Design review of the part built by this model. Coordinates are the model's own, in mm. A direction names the side the tool comes from. Coordinates: 2 decimals unless noted, no trailing zeros. Write each loop counter-clockwise with the first axis right and the second up, starting at its lowest first coordinate (ties: lowest second). Pieces come first, ordered by that corner, then holes.
Q1. For L1, parallel to X at y = 1.3, z = 9; L2, parallel to Z at x = -13, y = -3.75; L3, parallel to X at y = -0.05, z = 9, list the stretches that pass through material, from the lowest coordinate up.
Q2. For faces 1 (the flat face through (8, -4, -12.5)), 2 (the flat face through (0, 0, 0)), 3 (the flat face through (5.5, 1, -9)), list the 3-axis set-ups (+Z, -Z, +X, -X, +Y, -Y) from which the entire face can be reached by the end or side of a thin tool; tool diameter is ignored.
Q3. Take a section at A-A, the plane x = 0. Write out the cut boundary in (y, z).
Q4. The part is to be moulded in two halves that separate along Z. For faces 4 (the cylindrical face through (0.481, 0.816, 10.526)), 5 (the flat face through (0, 1, -2.25)), 6 (the flat face through (0, 2, 0)), say which applies: released by +Z, released by -Z, zero draft, split by the parting line, or undercut.
Q5. Take a section at D-D, the plane y = -4.75. Write out the cut boundary in (x, z).
Q6. Take a section at B-B, the plane y = 0.5. Write out the cut boundary in (x, z), plus the area to 3 significant figures.
Q7. Take a section at C-C, the plane x = -9. Write out the cut boundary in (y, z).
Q8. For pin 1 Ø0.6 at (x, y) = (1, 1) entering from -Z; pin 2 Ø4 at (x, z) = (18, 0.5) entering from -Y; pin 3 Ø5 at (y, z) = (-1.5, -10) entering from -X, all flat-tipped, find the tip position at first contact; note any pin that passes through.
from build123d import *

# Parameters (mm, degrees)
BOSS_EXTRUDE1_DEPTH = 2
BOSS_EXTRUDE2_START = 9.5
BOSS_EXTRUDE2_DEPTH = 9.5
CHAMFER1_SIZE       = 0.5
CHAMFER1_SIZE2      = 3
CHAMFER2_SIZE       = 1.083333
CHAMFER2_SIZE_2     = 6.5
SKETCH4_W           = 11
SKETCH4_H           = 10.25
CUT_EXTRUDE1_DEPTH  = 29.191310718
SKETCH5_R           = 1.6
CUT_EXTRUDE2_DEPTH  = 29.191310718


with BuildPart() as part:
    # Sketch1 → Boss-Extrude1 (new body)
    with BuildSketch(Plane(origin=(0, 0, 0), x_dir=(1, 0, 0), z_dir=(0, 1, 0))):
        with BuildLine():
            Line((-22.5, 0), (-10, 0))
            Line((-10, 0), (0, 0))
            Line((0, 0), (0, 12.5))
            Line((0, 12.5), (-10, 12.5))
            ThreePointArc((-10, 12.5), (-18.838834765, 8.838834765), (-22.5, 0))
        make_face()
        with BuildLine():
            Line((0, 0), (-10, 0))
            Line((-10, 0), (-22.5, 0))
            ThreePointArc((-22.5, 0), (-18.838834765, -8.838834765), (-10, -12.5))
            Line((-10, -12.5), (0, -12.5))
            Line((0, -12.5), (0, 0))
        make_face()
        with BuildLine():
            Line((0, 12.5), (0, 0))
            Line((0, 0), (10, 0))
            Line((10, 0), (22.5, 0))
            ThreePointArc((22.5, 0), (18.838834765, 8.838834765), (10, 12.5))
            Line((10, 12.5), (0, 12.5))
        make_face()
        with BuildLine():
            Line((10, 0), (0, 0))
            Line((0, 0), (0, -12.5))
            Line((0, -12.5), (10, -12.5))
            ThreePointArc((10, -12.5), (18.838834765, -8.838834765), (22.5, 0))
            Line((22.5, 0), (10, 0))
        make_face()
    extrude(amount=BOSS_EXTRUDE1_DEPTH)

    # Sketch2 → Boss-Extrude2 (add)
    with BuildSketch(Plane.XZ.offset(BOSS_EXTRUDE2_START)):
        with BuildLine():
            Line((-10, -12.5), (10, -12.5))
            ThreePointArc((10, -12.5), (22.5, 0), (10, 12.5))
            Line((10, 12.5), (-10, 12.5))
            ThreePointArc((-10, 12.5), (-22.5, 0), (-10, -12.5))
        make_face()
        with BuildLine():
            Line((-10, -11.5), (10, -11.5))
            ThreePointArc((10, -11.5), (21.5, 0), (10, 11.5))
            Line((10, 11.5), (-10, 11.5))
            ThreePointArc((-10, 11.5), (-21.5, 0), (-10, -11.5))
        make_face(mode=Mode.SUBTRACT)
    extrude(amount=-BOSS_EXTRUDE2_DEPTH)

    # Chamfer1
    chamfer1_edges = [part.edges().sort_by_distance(p)[0] for p in [
        (-21.5, -9.5, 0),
        (0, -9.5, -11.5),
        (21.5, -9.5, 0),
        (0, -9.5, 11.5),
    ]]
    chamfer1_side = [part.faces().sort_by_distance(p)[0] for p in [
        (0, -9.5, -11.985218493),
    ]]
    chamfer(chamfer1_edges, length=CHAMFER1_SIZE, length2=CHAMFER1_SIZE2, reference=chamfer1_side[0])

    # Chamfer2
    # the kernel refuses this chamfer: 6.5, 1.083333 mm, written as the material it adds along each edge
    with BuildSketch(Plane(origin=(10, 0, 0), x_dir=(0, 0, -1), z_dir=(-1, 0, 0))) as chamfer2_piece_1:
        Polygon((11.5 - CHAMFER2_SIZE, 0), (11.5, CHAMFER2_SIZE_2), (11.5, 0), align=None)
    revolve(axis=Axis((10, 0, 0), (0, -1, 0)), revolution_arc=180)
    with BuildSketch(Plane(origin=(10, 0, 11.5), x_dir=(0, 0.22206230346399594, -0.9750324781156083), z_dir=(-1, 0, 0))) as chamfer2_piece_2:
        Polygon((CHAMFER2_SIZE * 0.975032478116, CHAMFER2_SIZE * 0.222062303464), (-CHAMFER2_SIZE_2 * 0.222062303464, CHAMFER2_SIZE_2 * 0.975032478116), (0, 0), align=None)
    extrude(amount=20)
    with BuildSketch(Plane(origin=(-10, 0, -11.5), x_dir=(0, -0.9999799892692318, -0.006326220127935647), z_dir=(1, 0, 0))) as chamfer2_piece_3:
        Polygon((CHAMFER2_SIZE_2 * 0.999979989269, -CHAMFER2_SIZE_2 * 0.00632622012794), (-CHAMFER2_SIZE * 0.00632622012794, -CHAMFER2_SIZE * 0.999979989269), (0, 0), align=None)
    extrude(amount=20)
    with BuildSketch(Plane(origin=(-10, 0, 0), x_dir=(0, 0, 1), z_dir=(1, 0, 0))) as chamfer2_piece_4:
        Polygon((11.5, CHAMFER2_SIZE_2), (11.5 - CHAMFER2_SIZE, 0), (11.5, 0), align=None)
    revolve(axis=Axis((-10, 0, 0), (0, -1, 0)), revolution_arc=180)

    # Sketch4 → Cut-Extrude1 (cut, through all)
    with BuildSketch(Plane(origin=(0, 2, 0), x_dir=(1, 0, 0), z_dir=(0, 1, 0))):
        with Locations((0, 7.375)):
            Rectangle(SKETCH4_W, SKETCH4_H)
    extrude(amount=-CUT_EXTRUDE1_DEPTH, mode=Mode.SUBTRACT)

    # Sketch5 → Cut-Extrude2 (cut, through all)
    with BuildSketch(Plane(origin=(0, 2, 0), x_dir=(1, 0, 0), z_dir=(0, 1, 0))):
        with Locations(Location((0, -9, 0), (0, 0, 270))):
            Circle(SKETCH5_R)
    extrude(amount=-CUT_EXTRUDE2_DEPTH, mode=Mode.SUBTRACT)


solid = part.part
Responses:
1. L1: x = -18.67 to -1.6, 1.6 to 18.67
1. L2: z = -12.13 to -10.63, 10.63 to 12.13
1. L3: x = -18.67 to -15.26, 15.26 to 18.67
2. face 1: -Z, +X, -X, +Y, -Y
2. face 2: -Y
2. face 3: -Z, +Y, -Y
3. outline: (-9.5, 12) - (-1.1, 10.6) - (2, 10.6) - (2, 12.5) - (-9.5, 12.5) - close; (0, -2.25) - (2, -2.25) - (2, 7.4) - (0, 7.4) - close
4. face 4: undercut
4. face 5: released by -Z
4. face 6: zero draft
5. outline: (-10, -12.5) - (-5.5, -12.5) - (-5.5, -11.21) - (-10, -11.21) arc R11.21 cw to (-10, 11.21) - (10, 11.21) arc R11.21 cw to (10, -11.21) - (5.5, -11.21) - (5.5, -12.5) - (10, -12.5) arc R12.5 ccw to (10, 12.5) - (-10, 12.5) arc R12.5 ccw to start
6. outline: (-10, -12.5) - (-5.5, -12.5) - (-5.5, -2.25) - (5.5, -2.25) - (5.5, -12.5) - (10, -12.5) arc R12.5 ccw to (10, 12.5) - (-10, 12.5) arc R12.5 ccw to start; hole circle Ø3.2 at (0, 9)
6. area: 870 mm2
7. outline: (-9.5, -12.5) - (2, -12.5) - (2, 12.5) - (-9.5, 12.5) - (-9.5, 12) - (0, 10.42) - (0, -10.42) - (-9.5, -12) - close
8. pin 1: stops at z = -2.25
8. pin 2: stops at y = 0
8. pin 3: stops at x = -20
